```python
from build123d import *

# Parameters (mm, degrees)
BOSS_EXTRUDE1_START = -19.5
SKETCH1_R           = 1.95
BOSS_EXTRUDE1_DEPTH = 4
SKETCH2_W           = 10
SKETCH2_H           = 10
SKETCH2_R           = 1.525
BOSS_EXTRUDE2_DEPTH = 4
SKETCH2_3_R         = 1.525
CUT_EXTRUDE1_DEPTH  = 4
FILLET1_START       = -24
FILLET1_DEPTH       = 5
FILLET1_START_2     = -23.5
FILLET1_2_DEPTH     = 4


with BuildPart() as part:
    # Sketch1 → Boss-Extrude1 (new body)
    with BuildSketch(Plane(origin=(0, 0, 0), x_dir=(1, 0, 0), z_dir=(0, 1, 0)).offset(BOSS_EXTRUDE1_START)):
        with BuildLine():
            Line((43.9, 5), (-54.1, 5))
            ThreePointArc((-54.1, 5), (-59.1, 0), (-54.1, -5))
            Line((-54.1, -5), (43.9, -5))
            ThreePointArc((43.9, -5), (48.9, 0), (43.9, 5))
        make_face()
        with Locations(Location((43.9, 0, 0), (0, 0, 270))):
            Circle(SKETCH1_R, mode=Mode.SUBTRACT)
        with Locations(Location((-54.1, 0, 0), (0, 0, 270))):
            Circle(SKETCH1_R, mode=Mode.SUBTRACT)
    extrude(amount=-BOSS_EXTRUDE1_DEPTH)

    # Sketch2 → Boss-Extrude2 (add)
    # profile 1 of 4: a face of its own
    with BuildSketch(Plane(origin=(0, -19.5, 0), x_dir=(1, 0, 0), z_dir=(0, 1, 0))):
        with Locations((-40.1, -10)):
            Rectangle(SKETCH2_W, SKETCH2_H)
        with Locations(Location((-40.1, -10, 0), (0, 0, 270))):
            Circle(SKETCH2_R, mode=Mode.SUBTRACT)
    # profile 2 of 4: a face of its own
    with BuildSketch(Plane(origin=(0, -19.5, 0), x_dir=(1, 0, 0), z_dir=(0, 1, 0))):
        with Locations((-40.1, 10)):
            Rectangle(SKETCH2_W, SKETCH2_H)
        with Locations(Location((-40.1, 10, 0), (0, 0, 270))):
            Circle(SKETCH2_R, mode=Mode.SUBTRACT)
    # profile 3 of 4: a face of its own
    with BuildSketch(Plane(origin=(0, -19.5, 0), x_dir=(1, 0, 0), z_dir=(0, 1, 0))):
        with Locations((29.9, 10)):
            Rectangle(SKETCH2_W, SKETCH2_H)
        with Locations(Location((29.9, 10, 0), (0, 0, 270))):
            Circle(SKETCH2_R, mode=Mode.SUBTRACT)
    # profile 4 of 4: a face of its own
    with BuildSketch(Plane(origin=(0, -19.5, 0), x_dir=(1, 0, 0), z_dir=(0, 1, 0))):
        with Locations((29.9, -10)):
            Rectangle(SKETCH2_W, SKETCH2_H)
        with Locations(Location((29.9, -10, 0), (0, 0, 270))):
            Circle(SKETCH2_R, mode=Mode.SUBTRACT)
    extrude(amount=-BOSS_EXTRUDE2_DEPTH)

    # Sketch2<3> → Cut-Extrude1 (cut)
    with BuildSketch(Plane(origin=(0, -19.5, 0), x_dir=(1, 0, 0), z_dir=(0, 1, 0))):
        with Locations(Location((29.9, 0, 0), (0, 0, 270))):
            Circle(SKETCH2_3_R)
        with Locations(Location((-40.1, 0, 0), (0, 0, 270))):
            Circle(SKETCH2_3_R)
    extrude(amount=-CUT_EXTRUDE1_DEPTH, mode=Mode.SUBTRACT)

    # Fillet1: read off the stored shape, not the designer's step
    # Fillet1 outline → Fillet1 (cut)
    with BuildSketch(Plane(origin=(0, 0, 0), x_dir=(1, 0, 0), z_dir=(0, 1, 0)).offset(FILLET1_START)):
        with BuildLine():
            Line((34.9, -15), (34.9, -10))
            ThreePointArc((34.9, -10), (33.435533906, -13.535533906), (29.9, -15))
            Line((29.9, -15), (34.9, -15))
        make_face()
        with BuildLine():
            Line((-45.1, -15), (-40.1, -15))
            ThreePointArc((-40.1, -15), (-43.635533906, -13.535533906), (-45.1, -10))
            Line((-45.1, -10), (-45.1, -15))
        make_face()
        with BuildLine():
            Line((-35.1, -15), (-35.1, -10))
            ThreePointArc((-35.1, -10), (-36.564466094, -13.535533906), (-40.1, -15))
            Line((-40.1, -15), (-35.1, -15))
        make_face()
        with BuildLine():
            Line((24.9, -15), (29.9, -15))
            ThreePointArc((29.9, -15), (26.364466094, -13.535533906), (24.9, -10))
            Line((24.9, -10), (24.9, -15))
        make_face()
        with BuildLine():
            Line((34.9, 15), (29.9, 15))
            ThreePointArc((29.9, 15), (33.435533906, 13.535533906), (34.9, 10))
            Line((34.9, 10), (34.9, 15))
        make_face()
        with BuildLine():
            Line((24.9, 15), (24.9, 10))
            ThreePointArc((24.9, 10), (26.364466094, 13.535533906), (29.9, 15))
            Line((29.9, 15), (24.9, 15))
        make_face()
        with BuildLine():
            ThreePointArc((-45.1, 10), (-43.635533906, 13.535533906), (-40.1, 15))
            Line((-40.1, 15), (-45.1, 15))
            Line((-45.1, 15), (-45.1, 10))
        make_face()
        with BuildLine():
            ThreePointArc((-40.1, 15), (-36.564466094, 13.535533906), (-35.1, 10))
            Line((-35.1, 10), (-35.1, 15))
            Line((-35.1, 15), (-40.1, 15))
        make_face()
    extrude(amount=FILLET1_DEPTH, mode=Mode.SUBTRACT)

    # Fillet1 2 outline → Fillet1 2 (add)
    with BuildSketch(Plane(origin=(0, 0, 0), x_dir=(1, 0, 0), z_dir=(0, 1, 0)).offset(FILLET1_START_2)):
        with BuildLine():
            Line((34.9, -5), (34.9, -10))
            ThreePointArc((34.9, -10), (36.364466094, -6.464466094), (39.9, -5))
            Line((39.9, -5), (34.9, -5))
        make_face()
        with BuildLine():
            ThreePointArc((-50.1, -5), (-46.564466094, -6.464466094), (-45.1, -10))
            Line((-45.1, -10), (-45.1, -5))
            Line((-45.1, -5), (-50.1, -5))
        make_face()
        with BuildLine():
            ThreePointArc((-35.1, -10), (-33.635533906, -6.464466094), (-30.1, -5))
            Line((-30.1, -5), (-35.1, -5))
            Line((-35.1, -5), (-35.1, -10))
        make_face()
        with BuildLine():
            ThreePointArc((19.9, -5), (23.435533906, -6.464466094), (24.9, -10))
            Line((24.9, -10), (24.9, -5))
            Line((24.9, -5), (19.9, -5))
        make_face()
        with BuildLine():
            ThreePointArc((39.9, 5), (36.364466094, 6.464466094), (34.9, 10))
            Line((34.9, 10), (34.9, 5))
            Line((34.9, 5), (39.9, 5))
        make_face()
        with BuildLine():
            Line((-45.1, 5), (-45.1, 10))
            ThreePointArc((-45.1, 10), (-46.564466094, 6.464466094), (-50.1, 5))
            Line((-50.1, 5), (-45.1, 5))
        make_face()
        with BuildLine():
            Line((-35.1, 5), (-30.1, 5))
            ThreePointArc((-30.1, 5), (-33.635533906, 6.464466094), (-35.1, 10))
            Line((-35.1, 10), (-35.1, 5))
        make_face()
        with BuildLine():
            ThreePointArc((24.9, 10), (23.435533906, 6.464466094), (19.9, 5))
            Line((19.9, 5), (24.9, 5))
            Line((24.9, 5), (24.9, 10))
        make_face()
    extrude(amount=FILLET1_2_DEPTH)


solid = part.part
```
The listing builds one solid part. Answer for the finished solid, in the listing's coordinates (mm). A direction names the side the tool comes from. Give positions to 0.01 mm unless a question says otherwise; leave off trailing zeros. Loops run counter-clockwise (first coordinate to the right, second up) from the corner with the lowest first, then second, coordinate; pieces in that order, holes last. Notation, with made-up numbers: (16.5, -8.75) - (65.5, -8.75) arc R25 ccw to (65.5, 21.25) - close; hole circle Ø10 at (-38, -22.5). An arc over 180 degrees is marked (long way). Return JSON: item names as keys, results as strings. Group by question number.
1. Which of the six approach directions +Z, -Z, +X, -X, +Y, -Y give full straight-line access (tool end or side, diameter ignored) to faces 4 (the flat face through (-5, -21, 5)), 5 (the flat face through (-52, -21, -5)), 6 (the flat face through (42, -21, 5))?
2. Find section B-B (z = 0). Write down the section's boundary in (x, y) (3 decimals).
3. Find section D-D (x = 36). Write down the section's boundary in (y, z).
4. Find section C-C (x = -20). Write down the section's boundary in (y, z).
5. Straight lines are drawn through the part: line 1 (X direction, y = -20.75, z = 10) (3 decimals); line 2 (X direction, y = -21.05, z = 0) (3 decimals); line 3 (X direction, y = -22.65, z = 1.75). For each, find the intervals that lie inside material, in ascending order. Write a range as [from, to].
6. Find section A-A (y = -21.95). State how many separate pieces and enclosed holes the cut face has, then the cut area to 3 significant figures.
7. Given pin 1 Ø2 at (x, y) = (-5, -21.5) entering from -Z; pin 2 Ø2 at (x, y) = (-8, -21.5) entering from +Z; pin 3 Ø1.5 at (y, z) = (-21.5, 9) entering from +X, each flat-ended and moving along its own axis, determine where each tip first touches the part or whether it passes through.
8. Determine the mould class of faces 1 (the cylindrical face through (48.9, -21.5, 0.1)), 2 (the flat face through (-6, -19.5, 0)), 3 (the flat face through (-5, -21, -5)) for opening direction X: pulls with the +X half, pulls with the -X half, needs draft (parallel to the pull), parting line crosses it, or undercut.
Verdict:
{
 "1": {"face 4": "+Z, +Y, -Y", "face 5": "-Z, -X, +Y, -Y", "face 6": "+Z, +X, +Y, -Y"},
 "2": {"outline": "(-59.1, -23.5) - (-56.05, -23.5) - (-56.05, -19.5) - (-59.1, -19.5) - close; (-52.15, -23.5) - (-41.625, -23.5) - (-41.625, -19.5) - (-52.15, -19.5) - close; (-38.575, -23.5) - (28.375, -23.5) - (28.375, -19.5) - (-38.575, -19.5) - close; (31.425, -23.5) - (41.95, -23.5) - (41.95, -19.5) - (31.425, -19.5) - close; (45.85, -23.5) - (48.9, -23.5) - (48.9, -19.5) - (45.85, -19.5) - close"},
 "3": {"outline": "(-23.5, -6.87) - (-19.5, -6.87) - (-19.5, 6.87) - (-23.5, 6.87) - close"},
 "4": {"outline": "(-23.5, -5) - (-19.5, -5) - (-19.5, 5) - (-23.5, 5) - close"},
 "5": {"line 1": "x = [-45.1, -41.625], [-38.575, -35.1], [24.9, 28.375], [31.425, 34.9]", "line 2": "x = [-59.1, -56.05], [-52.15, -41.625], [-38.575, 28.375], [31.425, 41.95], [45.85, 48.9]", "line 3": "x = [-58.78, -54.96], [-53.24, 43.04], [44.76, 48.58]"},
 "6": {"separate pieces": "1", "enclosed holes": "8", "area": "1,390 mm^2"},
 "7": {"pin 1": "stops at z = -5", "pin 2": "stops at z = 5", "pin 3": "stops at x = 35.22"},
 "8": {"face 1": "pulls with the +X half", "face 2": "needs draft", "face 3": "undercut"}
}
